from build123d import *

# Parameters (mm, degrees)
SKETCH_1_R          = 2.5
SKETCH_1_R_2        = 23.57
EXTRUDE_1_DEPTH     = 2
CUT_EXTRUDE_1_DEPTH = 2


with BuildPart() as part:
    # 草图1 → 凸台-拉伸1 (new body)
    with BuildSketch(Plane.XY):
        Polygon((53.57, -53.57), (373.57, -23.57), (53.57, 6.43), (23.57, 326.43), (-6.43, 6.43), (-6.43, -53.57), align=None)
        Circle(SKETCH_1_R, mode=Mode.SUBTRACT)
        with Locations((47.14, 0)):
            Circle(SKETCH_1_R, mode=Mode.SUBTRACT)
        with Locations((0, -47.14)):
            Circle(SKETCH_1_R, mode=Mode.SUBTRACT)
        with Locations((47.14, -47.14)):
            Circle(SKETCH_1_R, mode=Mode.SUBTRACT)
        with Locations((23.57, -23.57)):
            Circle(SKETCH_1_R_2, mode=Mode.SUBTRACT)
    extrude(amount=EXTRUDE_1_DEPTH)

    # 草图2 → 切除-拉伸1 (cut)
    with BuildSketch(Plane.XY.offset(2)):
        Polygon((-1.767766953, 1.767766953), (-23.224943384, -19.689409478), (-48.141739781, -16.773526249), (-61.418914174, -41.57875584), (11.806639012, -99.639884024), (27.505819552, -70.309714354), (48.907766953, -48.907766953), (45.372233047, -45.372233047), (37.174466094, -53.57), (-6.43, -9.965533906), (1.767766953, -1.767766953), align=None)
        Polygon((45.372233047, 1.767766953), (27.505819552, -16.098646542), (32.100864157, -18.574669749), (48.907766953, -1.767766953), align=None)
    extrude(amount=-CUT_EXTRUDE_1_DEPTH, mode=Mode.SUBTRACT)


solid = part.part
Here's how the part is built. I have some questions about the finished solid (model axes, mm). A direction names the side the tool comes from. Give positions to 0.01 mm unless a question says otherwise; leave off trailing zeros. Order: outer loops, then holes, each group sorted by start corner. A loop starts at its lowest first (then second) coordinate and runs counter-clockwise, first axis right, second up. Notation, with made-up numbers: (61.5, -20) -> (110.5, -20) arc R12 cw to (110.5, 0) -> close; hole circle Ø4 at (81.25, -7). An arc over 180 degrees is marked (long way). Use a Markdown table: item, result. Add a question column.
Item 1: If we mould it in two halves opening along Y, with no side actions, what happens to faces 3 (the face through (38.78, 164.19, 0.99)), 4 (the face through (45.91, -31.08, 0.99)), 5 (the face through (211.33, -38.78, 0.99))? For each: pulls with the +Y half, pulls with the -Y half, needs draft (parallel to the pull), parting line crosses it, or undercut.
Item 2: Imagine slicing it at A-A on z = 1.3. Please give me the cut outline in (x, y).
Item 3: Imagine slicing it at B-B on x = 318. Please give me the cut outline in (y, z).
Item 4: Imagine slicing it at C-C on y = 271. Please give me the cut outline in (x, z).
Item 5: I need wall thicknesses on line 1 (X direction, y = 293.5, z = 1.1); line 2 (Y direction, x = 218.5, z = 0.6); line 3 (X direction, y = 12, z = 0.9). Which ranges of each line are inside material? Lowest first, please.
Item 6: For faces 1 (the face through (16.686, -1.028, 0.986)), 2 (the face through (215.81, -8.78, 0.99)), which set-ups out of +Z, -Z, +X, -X, +Y, -Y let a thin tool reach every point of the face, with its end or its side?
Data:
| question | item | result |
|---|---|---|
| 1 | face 3 | pulls with the +Y half |
| 1 | face 4 | undercut |
| 1 | face 5 | pulls with the -Y half |
| 2 | outline | (-6.43, -9.97) -> (0.86, -17.26) arc R23.57 cw to (38.37, -5.23) -> (45.37, 1.77) arc R2.5 cw to (48.91, -1.77) -> (41.91, -8.77) arc R23.57 cw to (29.88, -46.28) -> (37.17, -53.57) -> (45.37, -45.37) arc R2.5 cw to (48.91, -48.91) -> (44.25, -53.57) -> (53.57, -53.57) -> (373.57, -23.57) -> (53.57, 6.43) -> (23.57, 326.43) -> (-6.43, 6.43) -> (-6.43, -2.89) -> (-1.77, 1.77) arc R2.5 cw to (1.77, -1.77) -> close |
| 3 | outline | (-28.78, 0) -> (-18.36, 0) -> (-18.36, 2) -> (-28.78, 2) -> close |
| 4 | outline | (18.37, 0) -> (28.77, 0) -> (28.77, 2) -> (18.37, 2) -> close |
| 5 | line 1 | x = 20.48 to 26.66 |
| 5 | line 2 | y = -38.11 to -9.03 |
| 5 | line 3 | x = -5.91 to 53.05 |
| 6 | face 1 | +Z, -Z |
| 6 | face 2 | +Z, -Z, +X, +Y |
